```python
from build123d import *

# Parameters (mm, degrees)
F0_R     = 5.1
F1_DEPTH = 8
F3_D     = 2.5
F4_D     = 4.2
F4_DEPTH = 10.6
F4_TIP   = 1.2618073


with BuildPart() as f1:
    # F0 (on Front) → F1 (new body)
    with BuildSketch(Plane.XZ):
        with BuildLine():
            ThreePointArc((-7.80859375, 1.7395009766), (-5.6568542495, 5.6568542495), (-1.7395009766, 7.80859375))
            ThreePointArc((-1.7395009766, 7.80859375), (-1.3033535471, 9.1678054338), (0, 9.75))
            Line((0, 9.75), (0, 12.5))
            Line((0, 12.5), (-15, 12.5))
            Line((-15, 12.5), (-15, -12.5))
            Line((-15, -12.5), (0, -12.5))
            Line((0, -12.5), (0, -9.75))
            ThreePointArc((0, -9.75), (-1.3033535471, -9.1678054338), (-1.7395009766, -7.80859375))
            ThreePointArc((-1.7395009766, -7.80859375), (-5.6568542495, -5.6568542495), (-7.80859375, -1.7395009766))
            ThreePointArc((-7.80859375, -1.7395009766), (-9.75, 0), (-7.80859375, 1.7395009766))
        make_face()
        with BuildLine():
            ThreePointArc((1.7395009766, 7.80859375), (5.6568542495, 5.6568542495), (7.80859375, 1.7395009766))
            ThreePointArc((7.80859375, 1.7395009766), (9.1678054338, 1.3033535471), (9.75, 0))
            ThreePointArc((9.75, 0), (9.1678054338, -1.3033535471), (7.80859375, -1.7395009766))
            ThreePointArc((7.80859375, -1.7395009766), (5.6568542495, -5.6568542495), (1.7395009766, -7.80859375))
            ThreePointArc((1.7395009766, -7.80859375), (1.7473732728, -7.9041530099), (1.75, -8))
            ThreePointArc((1.75, -8), (1.2374368671, -9.2374368671), (0, -9.75))
            Line((0, -9.75), (0, -12.5))
            Line((0, -12.5), (15, -12.5))
            Line((15, -12.5), (15, 12.5))
            Line((15, 12.5), (0, 12.5))
            Line((0, 12.5), (0, 9.75))
            ThreePointArc((0, 9.75), (1.2374368671, 9.2374368671), (1.75, 8))
            ThreePointArc((1.75, 8), (1.7473732728, 7.9041530099), (1.7395009766, 7.80859375))
        make_face()
        with BuildLine():
            ThreePointArc((7.80859375, -1.7395009766), (6.25, 0), (7.80859375, 1.7395009766))
            ThreePointArc((7.80859375, 1.7395009766), (5.6568542495, 5.6568542495), (1.7395009766, 7.80859375))
            ThreePointArc((1.7395009766, 7.80859375), (0, 6.25), (-1.7395009766, 7.80859375))
            ThreePointArc((-1.7395009766, 7.80859375), (-5.6568542495, 5.6568542495), (-7.80859375, 1.7395009766))
            ThreePointArc((-7.80859375, 1.7395009766), (-6.6966464529, 1.1678054338), (-6.25, 0))
            ThreePointArc((-6.25, 0), (-6.6966464529, -1.1678054338), (-7.80859375, -1.7395009766))
            ThreePointArc((-7.80859375, -1.7395009766), (-5.6568542495, -5.6568542495), (-1.7395009766, -7.80859375))
            ThreePointArc((-1.7395009766, -7.80859375), (0, -6.25), (1.7395009766, -7.80859375))
            ThreePointArc((1.7395009766, -7.80859375), (5.6568542495, -5.6568542495), (7.80859375, -1.7395009766))
        make_face()
        Circle(F0_R, mode=Mode.SUBTRACT)
        with BuildLine():
            ThreePointArc((-1.7395009766, 7.80859375), (0, 8), (1.7395009766, 7.80859375))
            ThreePointArc((1.7395009766, 7.80859375), (1.7473732728, 7.9041530099), (1.75, 8))
            ThreePointArc((1.75, 8), (1.2374368671, 9.2374368671), (0, 9.75))
            ThreePointArc((0, 9.75), (-1.3033535471, 9.1678054338), (-1.7395009766, 7.80859375))
        make_face()
        with BuildLine():
            ThreePointArc((-7.80859375, -1.7395009766), (-8, 0), (-7.80859375, 1.7395009766))
            ThreePointArc((-7.80859375, 1.7395009766), (-9.75, 0), (-7.80859375, -1.7395009766))
        make_face()
        with BuildLine():
            ThreePointArc((-6.25, 0), (-6.6966464529, 1.1678054338), (-7.80859375, 1.7395009766))
            ThreePointArc((-7.80859375, 1.7395009766), (-8, 0), (-7.80859375, -1.7395009766))
            ThreePointArc((-7.80859375, -1.7395009766), (-6.6966464529, -1.1678054338), (-6.25, 0))
        make_face()
        with BuildLine():
            ThreePointArc((7.80859375, 1.7395009766), (7.9520044643, 0.875), (8, 0))
            ThreePointArc((8, 0), (7.9520044643, -0.875), (7.80859375, -1.7395009766))
            ThreePointArc((7.80859375, -1.7395009766), (9.1678054338, -1.3033535471), (9.75, 0))
            ThreePointArc((9.75, 0), (9.1678054338, 1.3033535471), (7.80859375, 1.7395009766))
        make_face()
        with BuildLine():
            ThreePointArc((7.80859375, -1.7395009766), (7.9520044643, -0.875), (8, 0))
            ThreePointArc((8, 0), (7.9520044643, 0.875), (7.80859375, 1.7395009766))
            ThreePointArc((7.80859375, 1.7395009766), (6.25, 0), (7.80859375, -1.7395009766))
        make_face()
        with BuildLine():
            ThreePointArc((-1.7395009766, -7.80859375), (0, -8), (1.7395009766, -7.80859375))
            ThreePointArc((1.7395009766, -7.80859375), (0, -6.25), (-1.7395009766, -7.80859375))
        make_face()
        with BuildLine():
            ThreePointArc((1.75, -8), (1.7473732728, -7.9041530099), (1.7395009766, -7.80859375))
            ThreePointArc((1.7395009766, -7.80859375), (0, -8), (-1.7395009766, -7.80859375))
            ThreePointArc((-1.7395009766, -7.80859375), (-1.3033535471, -9.1678054338), (0, -9.75))
            ThreePointArc((0, -9.75), (1.2374368671, -9.2374368671), (1.75, -8))
        make_face()
        with BuildLine():
            ThreePointArc((-1.7395009766, 7.80859375), (0, 6.25), (1.7395009766, 7.80859375))
            ThreePointArc((1.7395009766, 7.80859375), (0, 8), (-1.7395009766, 7.80859375))
        make_face()
    extrude(amount=F1_DEPTH)

    # F3 (through all)
    with Locations(Plane(origin=(0, 0, 0), x_dir=(1, 0, 0), z_dir=(0, 1, 0))):
        with Locations((0, -8), (8, 0), (-8, 0), (0, 8)):
            Hole(F3_D / 2)

    # F4
    with Locations(Plane.XY.offset(12.5)):
        with Locations((-10, -4), (10, -4)):
            Hole(F4_D / 2, depth=F4_DEPTH)
            with Locations((0, 0, -(F4_DEPTH + F4_TIP / 2))):  # 118° drill point
                Cone(0, F4_D / 2, F4_TIP, mode=Mode.SUBTRACT)


solid = f1.part
```
Read the model definition and answer for the solid it produces. Units are mm, in the model's axes. A direction names the side the tool comes from. Give positions to 0.01 mm unless a question says otherwise; leave off trailing zeros. Order: outer loops, then holes, each group sorted by start corner. A loop starts at its lowest first (then second) coordinate and runs counter-clockwise, first axis right, second up.
(1) Find section B-B (x = 0). Give the vertices of the cut face in (y, z).
(2) Find section A-A (z = -8). Give the vertices of the cut face in (x, y).
(3) Straight lines are drawn through the part: L1, parallel to X at y = -4, z = 9.75; L2, parallel to Z at x = 0, y = -4.5; L3, parallel to Y at x = -10, z = 5.5. For each, find the intervals that lie inside material, in ascending order.
(4) Given pin 1 (2 mm diameter, centred on x = -8, z = 0, fed in from -Y) (3 decimals); pin 2 (2.5 mm diameter, centred on x = -10, y = -4, fed in from +Z), each flat-ended and moving along its own axis, determine where each tip first touches the part or whether it passes through.
(5) Find section D-D (y = -7.5). Give the vertices of the cut face in (x, z), plus the area to 3 significant figures.
(6) Find section C-C (z = 8.75). Give the vertices of the cut face in (x, y).
(7) For a pull along Z with two mould halves and no side action, classify faces 3 (the flat face through (15, -4, 0)), 4 (the conical face through (9.636, -3.984, 0.857)), 5 (the cylindrical face through (2.4, -3.9, -4.5)) as released by +Z, released by -Z, zero draft, split by the parting line, or undercut.
(8) For faces 1 (the cylindrical face through (11.666, -5.278, 7.126)), 2 (the cylindrical face through (-6.75, -4.06, -0.05)), determine the directions among +Z, -Z, +X, -X, +Y, -Y from which every point of the face is accessible in a straight line to the end or side of a thin tool.
Result sheet:
1. outline: (-8, -12.5) - (0, -12.5) - (0, -9.25) - (-8, -9.25) - close; (-8, -6.75) - (0, -6.75) - (0, -5.1) - (-8, -5.1) - close; (-8, 5.1) - (0, 5.1) - (0, 6.75) - (-8, 6.75) - close; (-8, 9.25) - (0, 9.25) - (0, 12.5) - (-8, 12.5) - close
2. outline: (-15, -8) - (-1.25, -8) - (-1.25, 0) - (-15, 0) - close; (1.25, -8) - (15, -8) - (15, 0) - (1.25, 0) - close
3. L1: x = -15 to -12.1, -7.9 to 7.9, 12.1 to 15
3. L2: z = -12.5 to -9.25, -6.75 to -5.1, 5.1 to 6.75, 9.25 to 12.5
3. L3: y = -8 to -6.1, -1.9 to 0
4. pin 1: passes through
4. pin 2: stops at z = 1.39
5. outline: (-15, -12.5) - (15, -12.5) - (15, 12.5) - (-15, 12.5) - close; hole circle Ø2.5 at (-8, 0); hole circle Ø10.2 at (0, 0); hole circle Ø2.5 at (0, -8); hole circle Ø2.5 at (0, 8); hole circle Ø2.5 at (8, 0)
5. area: 649 mm2
6. outline: (-15, -8) - (-1, -8) - (-1, 0) - (-15, 0) - close; (1, -8) - (15, -8) - (15, 0) - (1, 0) - close; hole circle Ø4.2 at (-10, -4); hole circle Ø4.2 at (10, -4)
7. face 3: zero draft
7. face 4: released by +Z
7. face 5: undercut
8. face 1: +Z
8. face 2: +Y, -Y
